Drawing for the job (mm, zero at the part's lowest x, y, z). Round coordinates to 2 decimals unless told otherwise and drop trailing zeros. Write each loop counter-clockwise with the first axis right and the second up, starting at its lowest first coordinate (ties: lowest second). Pieces come first, ordered by that corner, then holes. Notation, with made-up numbers: M 1,14 L 11,14 A10 cw 11,27 Z; hole C -35,-34 d4. An arc over 180 degrees is marked long. Use a Markdown table: item, result. Add a question column.
1) Drop a flat-ended pin along its axis: P1, Ø2, axis at x = 22, z = 13.5, coming from the -Y side. Give the stop position or say it passes through.
2) Slice it at B-B on x = 33. Write the cut outline in (y, z).
3) Two-plate mould, pull along X, no slides. Class the marked faces 1, 2, 3 and 4: released by +X, released by -X, zero draft, split by the parting line, or undercut.
4) Wall check: probe 1 along X at (y, z) = (8, 6.75); probe 2 along X at (y, z) = (26, 9.25); probe 3 along Y at (x, z) = (35, 10). Give the ranges that are in metal, low to high.
5) Slice it at C-C on z = 12. Write the cut outline in (x, y) (3 decimals), plus the area to 3 significant figures.
6) Slice it at A-A on y = 2. Write the cut outline in (x, z), plus the area to 3 significant figures.
7) Slice it at D-D on x = 28.5. Write the cut outline in (y, z).
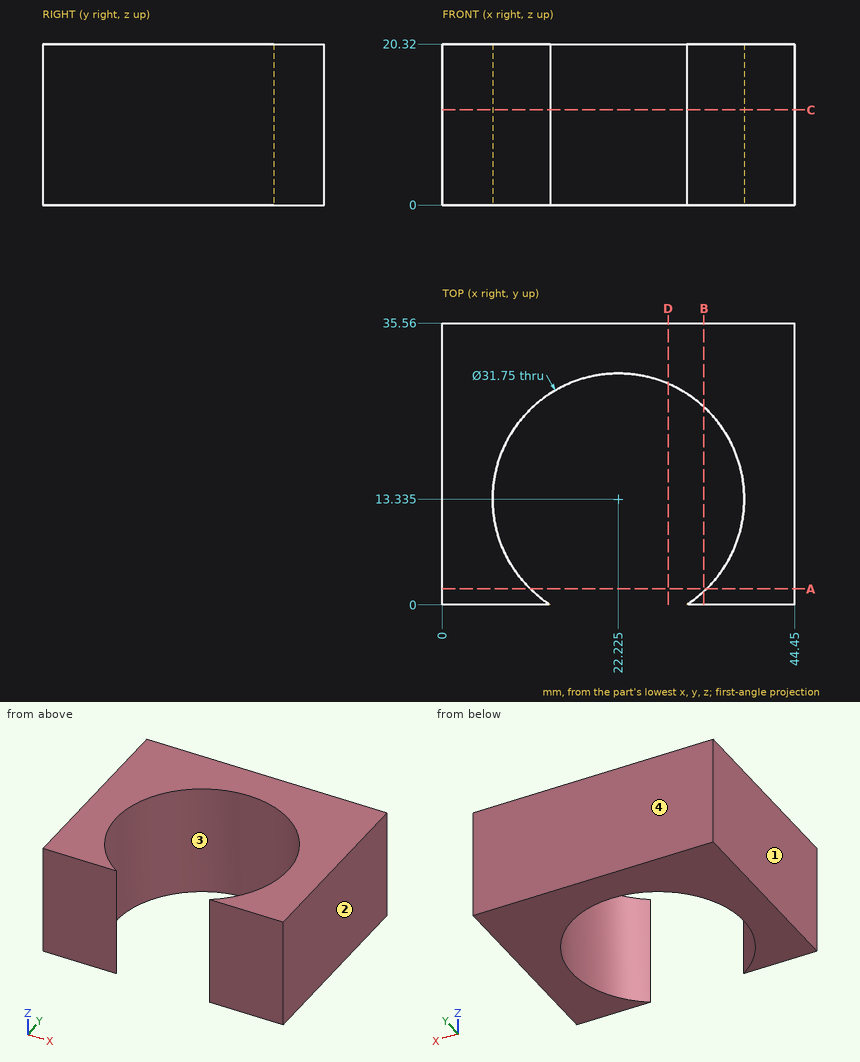
Entries:
| question | item | result |
|---|---|---|
| 1 | P1 | stops at y = 29.16 |
| 2 | outline | M 0,0 L 1.68,0 L 1.68,20.32 L 0,20.32 Z; M 24.99,0 L 35.56,0 L 35.56,20.32 L 24.99,20.32 Z |
| 3 | face 1 | released by -X |
| 3 | face 2 | released by +X |
| 3 | face 3 | undercut |
| 3 | face 4 | zero draft |
| 4 | probe 1 | x = 0 to 7.27, 37.18 to 44.45 |
| 4 | probe 2 | x = 0 to 12.65, 31.8 to 44.45 |
| 4 | probe 3 | y = 0 to 3.91, 22.76 to 35.56 |
| 5 | outline | M 0,0 L 13.611,0 A15.875 cw long 30.839,0 L 44.45,0 L 44.45,35.56 L 0,35.56 Z |
| 5 | area | 819 mm^2 |
| 6 | outline | M 0,0 L 11.11,0 L 11.11,20.32 L 0,20.32 Z; M 33.34,0 L 44.45,0 L 44.45,20.32 L 33.34,20.32 Z |
| 6 | area | 452 mm^2 |
| 7 | outline | M 27.92,0 L 35.56,0 L 35.56,20.32 L 27.92,20.32 Z |
